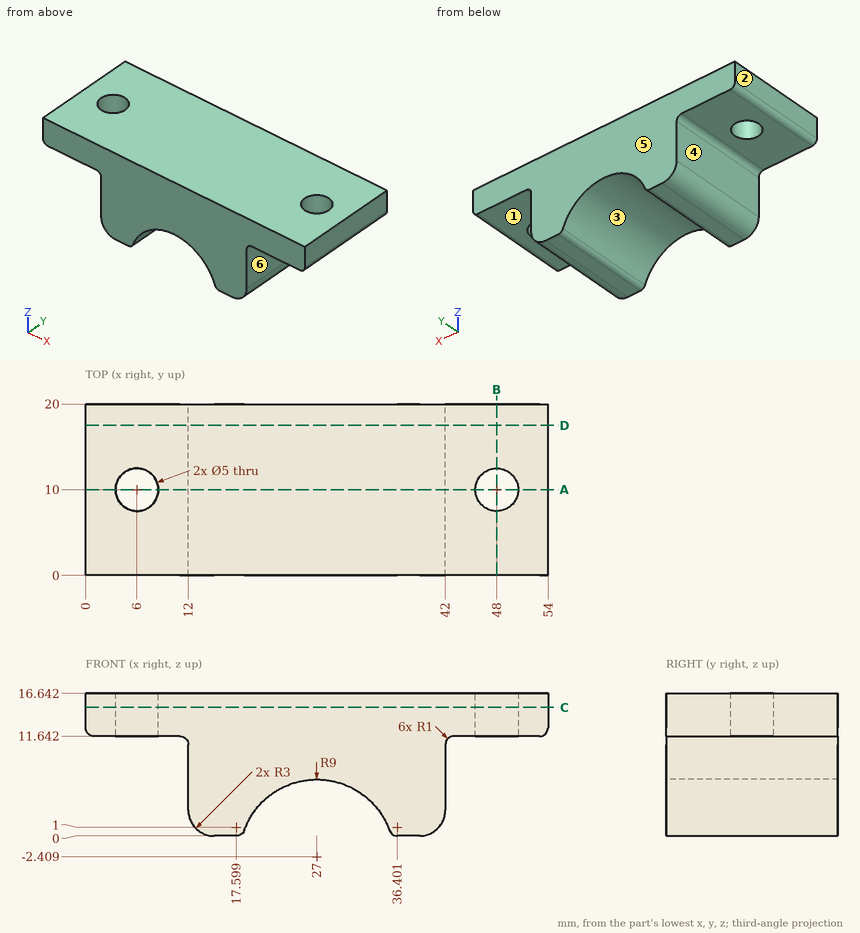
Input: dimensioned drawing with shaded views. Units: mm. Origin: part minimum x, y, z. A direction names the side the tool comes from. Round coordinates to 2 decimals unless told otherwise and drop trailing zeros. Loops run counter-clockwise (first coordinate to the right, second up) from the corner with the lowest first, then second, coordinate; pieces in that order, holes last. Notation, with made-up numbers: (81, -4) -> (95, -4) arc R21 cw to (95, 27) -> close; hole circle Ø3 at (9.5, 77.5). An arc over 180 degrees is marked (long way). Answer as a JSON object with one key per item and string values. Group by question number.
1) Section query B-B on x = 48. Output: boundary loops of the cut face in (y, z).
2) Draft query along X for the marked faces 1, 2 and 3. Return one class per face: +X half, -X half, draft (parallel to the pull), parting line (faces both ways), or undercut.
3) Reachability of the marked faces 4, 5 and 6 from +Z, -Z, +X, -X, +Y, -Y: full face, straight path, thin tool, end or side. Return the list, or none.
4) Section query A-A on y = 10. Output: boundary loops of the cut face in (x, z).
5) Pin query (flat end, axial travel): pin 1 (2.5 mm diameter, centred on y = 11.5, z = 8.5, fed in from -X); pin 2 (6.5 mm diameter, centred on x = 6, y = 10, fed in from +Z); pin 3 (2.5 mm diameter, centred on y = 8, z = 7, fed in from +X); pin 4 (8 mm diameter, centred on x = 50, y = 10.5, fed in from -Z). Return the tip coordinate at first contact, or that it passes through.
6) Ray query, L1, parallel to Y at x = 6, z = 14.9; L2, parallel to Z at x = 8, y = 4; L3, parallel to X at y = 10, z = 5. Return the intervals inside material, ascending.
7) Section query C-C on z = 15. Output: boundary loops of the cut face in (x, y).
8) Section query D-D on y = 17.5. Output: boundary loops of the cut face in (x, z).
Reply:
{
 "1": {"outline": "(0, 11.64) -> (7.5, 11.64) -> (7.5, 16.64) -> (0, 16.64) -> close; (12.5, 11.64) -> (20, 11.64) -> (20, 16.64) -> (12.5, 16.64) -> close"},
 "2": {"face 1": "draft", "face 2": "-X half", "face 3": "undercut"},
 "3": {"face 4": "-Z, -X, +Y, -Y", "face 5": "+Z, -Z, +X, -X, +Y", "face 6": "-Z, +X, +Y, -Y"},
 "4": {"outline": "(0, 12.64) arc R1 ccw to (1, 11.64) -> (3.5, 11.64) -> (3.5, 16.64) -> (0, 16.64) -> close; (8.5, 11.64) -> (11, 11.64) arc R1 cw to (12, 10.64) -> (12, 3) arc R3 ccw to (15, 0) -> (17.6, 0) arc R1 ccw to (18.54, 0.66) arc R9 cw to (35.46, 0.66) arc R1 ccw to (36.4, 0) -> (39, 0) arc R3 ccw to (42, 3) -> (42, 10.64) arc R1 cw to (43, 11.64) -> (45.5, 11.64) -> (45.5, 16.64) -> (8.5, 16.64) -> close; (50.5, 11.64) -> (53, 11.64) arc R1 ccw to (54, 12.64) -> (54, 16.64) -> (50.5, 16.64) -> close"},
 "5": {"pin 1": "stops at x = 12", "pin 2": "stops at z = 16.64", "pin 3": "stops at x = 42", "pin 4": "stops at z = 11.64"},
 "6": {"L1": "y = 0 to 7.5, 12.5 to 20", "L2": "z = 11.64 to 16.64", "L3": "x = 12 to 21.89, 32.11 to 42"},
 "7": {"outline": "(0, 0) -> (54, 0) -> (54, 20) -> (0, 20) -> close; hole circle Ø5 at (6, 10); hole circle Ø5 at (48, 10)"},
 "8": {"outline": "(0, 12.64) arc R1 ccw to (1, 11.64) -> (11, 11.64) arc R1 cw to (12, 10.64) -> (12, 3) arc R3 ccw to (15, 0) -> (17.6, 0) arc R1 ccw to (18.54, 0.66) arc R9 cw to (35.46, 0.66) arc R1 ccw to (36.4, 0) -> (39, 0) arc R3 ccw to (42, 3) -> (42, 10.64) arc R1 cw to (43, 11.64) -> (53, 11.64) arc R1 ccw to (54, 12.64) -> (54, 16.64) -> (0, 16.64) -> close"}
}
